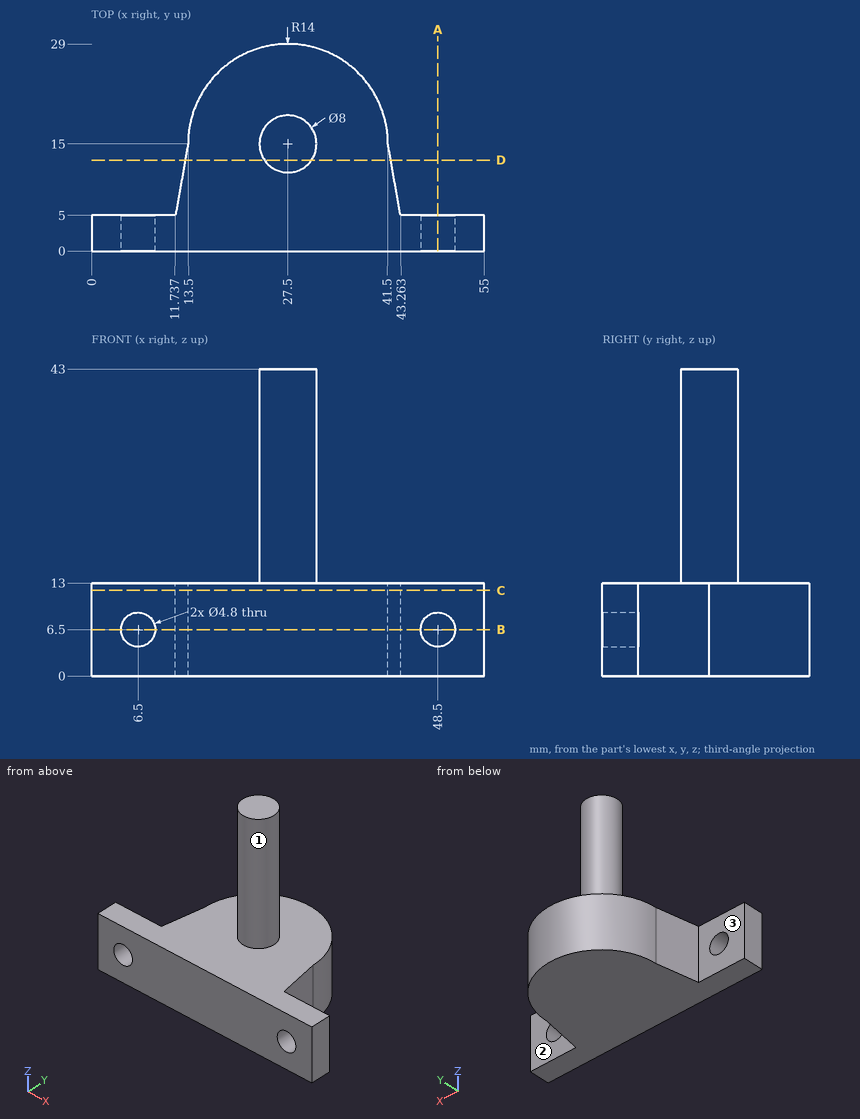
Job drawing, mm, ordinate dimensions from the low corner. One solid piece. A direction names the side the tool comes from. Give positions to 0.01 mm unless a question says otherwise; leave off trailing zeros. Loops run counter-clockwise (first coordinate to the right, second up) from the corner with the lowest first, then second, coordinate; pieces in that order, holes last. Notation, with made-up numbers: M 2.25,-12.5 L 52.25,-12.5 A16 cw 52.25,15.5 Z; hole C 44,5 d3. An arc over 180 degrees is marked long. Use one line per item in the form item = value.
Item 1: Drill centre lines: L1, parallel to Z at x = 6.5, y = 1.55; L2, parallel to Y at x = 9.5, z = 8; L3, parallel to Z at x = 41.5, y = 13.5. Where is each one in solid material? Low to high.
Filled in:
L1 = 0 to 4.1, 8.9 to 13
L2 = 0 to 5
L3 = 0 to 13
Item 2: Which spindle directions (+Z, -Z, +X, -X, +Y, -Y) get a long thin tool onto all of the face, cutting with end or side? Do the marked faces 1, 2 and 3. Say none if no direction does.
Filled in:
face_1 = +Z
face_2 = +Z, -Z, +X, +Y
face_3 = +Z, -Z, -X, +Y
Item 3: Slice it at B-B on z = 6.5. List the corners of the cut face in (x, y).
Filled in:
outline = M 0,0 L 4.1,0 L 4.1,5 L 0,5 Z; M 8.9,0 L 46.1,0 L 46.1,5 L 43.26,5 L 41.5,15 A14 ccw 13.5,15 L 11.74,5 L 8.9,5 Z; M 50.9,0 L 55,0 L 55,5 L 50.9,5 Z
Item 4: Slice it at C-C on z = 12. List the corners of the cut face in (x, y).
Filled in:
outline = M 0,0 L 55,0 L 55,5 L 43.26,5 L 41.5,15 A14 ccw 13.5,15 L 11.74,5 L 0,5 Z
Item 5: Slice it at D-D on y = 12.75. List the corners of the cut face in (x, z), and give its area (3 significant figures).
Filled in:
outline = M 13.1,0 L 41.9,0 L 41.9,13 L 30.81,13 L 30.81,43 L 24.19,43 L 24.19,13 L 13.1,13 Z
area = 573 mm^2
Item 6: Flat gauge pins, fed straight in: pin 1 Ø8 at (x, y) = (15.5, 19) entering from +Z; pin 2 Ø6 at (x, z) = (46.5, 4) entering from +Y; pin 3 Ø5 at (y, z) = (13.5, 23.5) entering from -X. Where does each tip first touch, or does it go through?
Filled in:
pin_1 = 13
pin_2 = 5
pin_3 = 23.5
Item 7: Slice it at A-A on x = 48.5. List the corners of the cut face in (y, z), and give its area (3 significant figures).
Filled in:
outline = M 0,0 L 5,0 L 5,4.1 L 0,4.1 Z; M 0,8.9 L 5,8.9 L 5,13 L 0,13 Z
area = 41.0 mm^2
